Drawing for the job (mm, zero at the part's lowest x, y, z). Give positions to 0.01 mm unless a question says otherwise; leave off trailing zeros.
1) Flat gauge pin, fed straight in: P1, Ø4, axis at y = 31, z = 10, coming from the -X side. Where does the tip first touch, or does it go through?
2) Wall check: line 1 (X direction, y = 40, z = 20) (1 decimal); line 2 (Y direction, x = 24, z = 20.25) (1 decimal). Give the ranges that are in metal, low to high.
3) Two-plate mould, pull along X, no slides. Class the marked faces 1, 2 and 3: +X half, -X half, draft (parallel to the pull), parting line (faces both ways), or undercut.
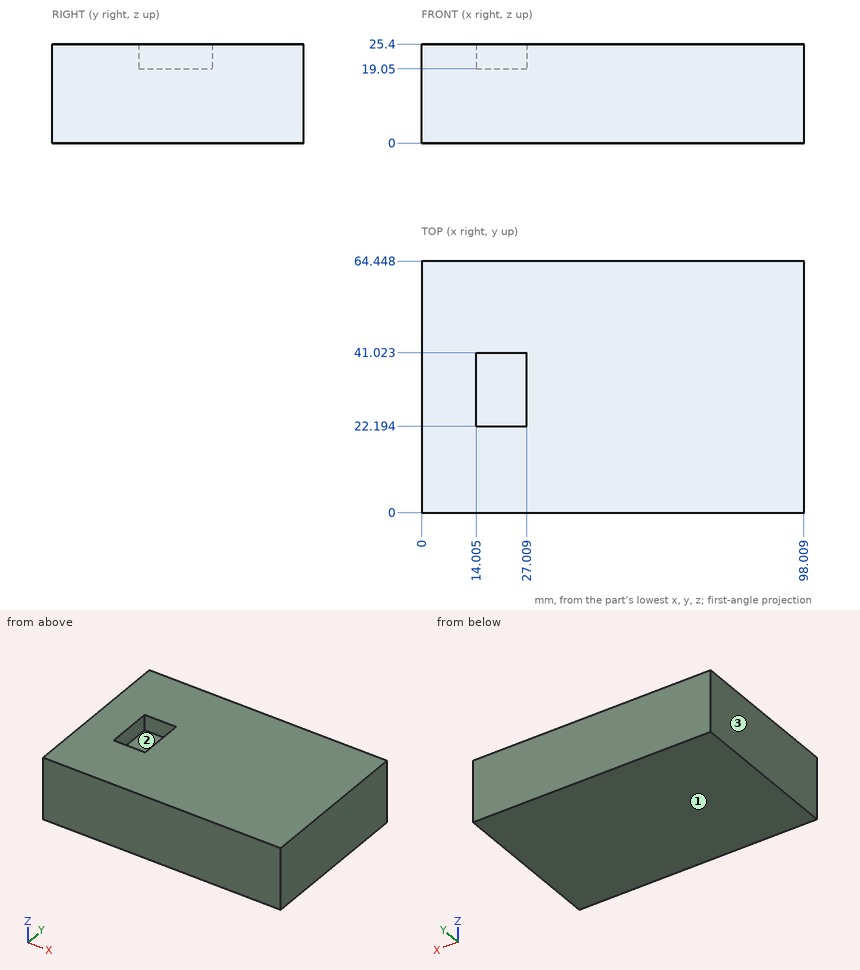
Findings below:
1. P1: stops at x = 0
2. line 1: x = 0 to 14, 27 to 98
2. line 2: y = 0 to 22.2, 41 to 64.4
3. face 1: draft
3. face 2: undercut
3. face 3: -X half
